```python
from build123d import *

# Parameters (mm, degrees)
SKETCH_2_R      = 2.5
EXTRUDE_1_DEPTH = 5
SKETCH_5_R      = 2.25
SKETCH_5_R_2    = 2.5
EXTRUDE_4_DEPTH = 10
SKETCH_6_R      = 2.25
EXTRUDE_5_DEPTH = 10


with BuildPart() as part:
    # 草圖2 → 填料-伸長1 (new body)
    with BuildSketch(Plane(origin=(0, 0, 0), x_dir=(1, 0, 0), z_dir=(0, 1, 0))):
        with BuildLine():
            Line((-32.334666667, 2.471706203), (-16.48, 17.447337906))
            ThreePointArc((-16.48, 17.447337906), (24, 0), (-16.48, -17.447337906))
            Line((-16.48, -17.447337906), (-32.334666667, -2.471706203))
            ThreePointArc((-32.334666667, -2.471706203), (-33.4, 0), (-32.334666667, 2.471706203))
        make_face()
        with Locations(Location((0, 0, 0), (0, 0, 270))):
            Circle(SKETCH_2_R, mode=Mode.SUBTRACT)
    extrude(amount=EXTRUDE_1_DEPTH)

    # 草圖5 → 填料-伸長4 (add)
    # profile 1 of 2: a face of its own
    with BuildSketch(Plane(origin=(0, 5, 0), x_dir=(1, 0, 0), z_dir=(0, 1, 0))):
        with Locations(Location((-30, 0, 0), (0, 0, 90))):
            Circle(SKETCH_5_R)
    # profile 2 of 2: a face of its own
    with BuildSketch(Plane(origin=(0, 5, 0), x_dir=(1, 0, 0), z_dir=(0, 1, 0))):
        with BuildLine():
            ThreePointArc((-20.773318517, -12.019535673), (24, 0), (-20.773318517, 12.019535673))
            ThreePointArc((-20.773318517, 12.019535673), (-16.277495404, 0), (-20.773318517, -12.019535673))
        make_face()
        with Locations(Location((0, 0, 0), (0, 0, 270))):
            Circle(SKETCH_5_R_2, mode=Mode.SUBTRACT)
    extrude(amount=EXTRUDE_4_DEPTH)

    # 草圖6 → 填料-伸長5 (add)
    with BuildSketch(Plane(origin=(0, 15, 0), x_dir=(1, 0, 0), z_dir=(0, 1, 0))):
        with Locations(Location((-30, 0, 0), (0, 0, 90))):
            Circle(SKETCH_6_R)
    extrude(amount=EXTRUDE_5_DEPTH)


solid = part.part
```
Here's how the part is built. I have some questions about the finished solid (model axes, mm). A direction names the side the tool comes from. Give positions to 0.01 mm unless a question says otherwise; leave off trailing zeros. Order: outer loops, then holes, each group sorted by start corner. A loop starts at its lowest first (then second) coordinate and runs counter-clockwise, first axis right, second up. Notation, with made-up numbers: (64, -23) - (120, -23) arc R8 cw to (120, -12) - close; hole circle Ø10 at (-20.75, 25). An arc over 180 degrees is marked (long way). Answer as a JSON object with one key per item and string values. Group by question number.
Item 1: If we section it at C-C on y = 6.25: Please give me the cut outline in (x, z).
Item 2: If we section it at D-D on y = 2.25: Please give me the cut outline in (x, z), and give its area (3 significant figures).
Item 3: If we mould it in two halves opening along X, with no side actions, what happens to faces 3 (the cylindrical face through (-33.4, 2.5, 0)), 4 (the cylindrical face through (-31.897, 14.86, -1.21)), 5 (the flat face through (6, 15, 0))? For each: pulls with the +X half, pulls with the -X half, needs draft (parallel to the pull), parting line crosses it, or undercut.
Item 4: If we section it at A-A on z = 0: Please give me the cut outline in (x, y), and give its area (3 significant figures).
Item 5: For P1, Ø8, axis at x = -22, z = 14.5, coming from the +Y side; P2, Ø5, axis at y = 7.5, z = -3, coming from the -X side; P3, Ø1, axis at y = 14.5, z = -18.5, coming from the +X side, each with a flat end and sliding along its axis, tell me the tip position at first contact or that it passes through.
Item 6: Which directions (+Z, -Z, +X, -X, +Y, -Y) give clear straight access to the entire face, cutting with the end or side of a thin tool? Please do faces 1 (the cylindrical face through (-2.44, 7.4, -0.54)), 2 (the flat face through (-23, 5, 0)).
Item 7: Please list where these lines run through material, in increasing order: probe 1 along Y at (x, z) = (-21, -10.5); probe 2 along Y at (x, z) = (-4, 15); probe 3 along X at (y, z) = (8.5, 10).
Item 8: If we section it at B-B on x = 0: Please give me the cut outline in (y, z), and give its area (3 significant figures).
Result set:
{
 "1": {"outline": "circle Ø4.5 at (-30, 0); (-20.77, -12.02) arc R24 ccw (long way) to (-20.77, 12.02) arc R18.31 cw to start; hole circle Ø5 at (0, 0)"},
 "2": {"outline": "(-32.33, -2.47) - (-16.48, -17.45) arc R24 ccw (long way) to (-16.48, 17.45) - (-32.33, 2.47) arc R3.4 ccw to start; hole circle Ø5 at (0, 0)", "area": "1,930 mm²"},
 "3": {"face 3": "pulls with the -X half", "face 4": "undercut", "face 5": "needs draft"},
 "4": {"outline": "(-33.4, 0) - (-2.5, 0) - (-2.5, 15) - (-16.28, 15) - (-16.28, 5) - (-27.75, 5) - (-27.75, 25) - (-32.25, 25) - (-32.25, 5) - (-33.4, 5) - close; (2.5, 0) - (24, 0) - (24, 15) - (2.5, 15) - close", "area": "705 mm²"},
 "5": {"P1": "y = 15", "P2": "x = -32.19", "P3": "x = 15.87"},
 "6": {"face 1": "+Y, -Y", "face 2": "+Y"},
 "7": {"probe 1": "0 to 5", "probe 2": "0 to 15", "probe 3": "-19.25 to 21.82"},
 "8": {"outline": "(0, -24) - (15, -24) - (15, -2.5) - (0, -2.5) - close; (0, 2.5) - (15, 2.5) - (15, 24) - (0, 24) - close", "area": "645 mm²"}
}
